Read the model definition and answer for the solid it produces. Units are mm, in the model's axes. Face numbers are marked on the shaded views. Give positions to 0.01 mm unless a question says otherwise; leave off trailing zeros. Order: outer loops, then holes, each group sorted by start corner. A loop starts at its lowest first (then second) coordinate and runs counter-clockwise, first axis right, second up. Notation, with made-up numbers: (64, 22) -> (95, 22) arc R27 ccw to (95, 52) -> close; hole circle Ø3 at (22.25, 17). An arc over 180 degrees is marked (long way). Answer as CSV lines item,"result". Start each with the question number.
1) A flat-ended cylindrical pin translates along its axis: pin 1 Ø16 at (x, y) = (45, 35) entering from +Z. Find the tip coordinate at first contact, or state that the pin passes through.
2) Find section C-C (x = 82). Determine the outline of the cut face in (y, z).
3) Find section D-D (y = 37). Determine the outline of the cut face in (x, z), and give its area (3 significant figures).
4) Find section B-B (y = 65). Determine the outline of the cut face in (x, z), and give its area (3 significant figures).
5) Find section A-A (x = 45). Determine the outline of the cut face in (y, z).
6) Straight lines are drawn through the part: L1, parallel to X at y = 7.5, z = 8; L2, parallel to Y at x = 45, z = 2.45; L3, parallel to Y at x = 45, z = 12.5. For each, find the intervals that lie inside material, in ascending order. Write a range as from..to.
7) The mould has two halves that part along Y. Classify the marked faces 1, 2, 3 and 4: +Y half, -Y half, draft (parallel to the pull), parting line (faces both ways), or undercut.
```python
from build123d import *

# Parameters (mm, degrees)
F0_W           = 90
F0_H           = 15
F4_D           = 8.8
F6_D           = 11
F6_CBORE_D     = 20
F6_CBORE_DEPTH = 12


with BuildPart() as f2:
    # F2: sweep along a path in F1
    with BuildLine(Plane.YZ) as f2_path:
        Line((0, 0), (70, 0))
    # F0 (on Front) → F2 (sweep)
    with BuildSketch(Plane.XZ):
        with Locations((45, 7.5)):
            Rectangle(F0_W, F0_H)
    sweep(path=f2_path.line)

    # F4 (through all)
    with Locations(Plane.XY.offset(15)):
        with Locations((8, 62), (82, 62), (82, 8), (8, 8)):
            Hole(F4_D / 2)

    # F6 (through all)
    with Locations(Plane.XY.offset(15)):
        with Locations((45, 35)):
            CounterBoreHole(F6_D / 2, F6_CBORE_D / 2, F6_CBORE_DEPTH)


solid = f2.part
```
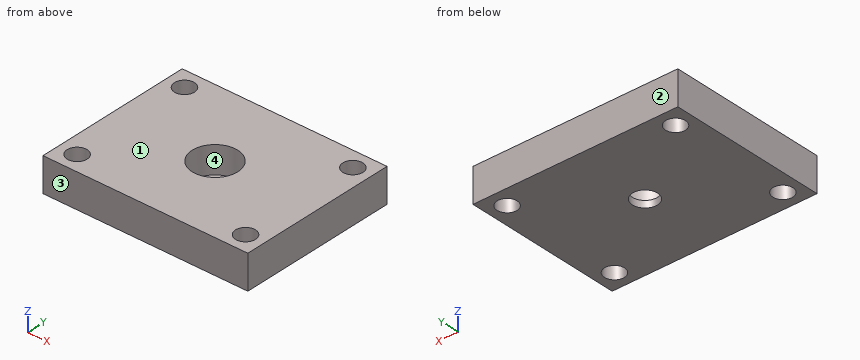
Findings below:
1,pin 1,"z = 3"
2,outline,"(0, 0) -> (3.6, 0) -> (3.6, 15) -> (0, 15) -> close; (12.4, 0) -> (57.6, 0) -> (57.6, 15) -> (12.4, 15) -> close; (66.4, 0) -> (70, 0) -> (70, 15) -> (66.4, 15) -> close"
3,outline,"(0, 0) -> (39.88, 0) -> (39.88, 3) -> (35.2, 3) -> (35.2, 15) -> (0, 15) -> close; (50.12, 0) -> (90, 0) -> (90, 15) -> (54.8, 15) -> (54.8, 3) -> (50.12, 3) -> close"
3,area,"1,080 mm²"
4,outline,"(0, 0) -> (4.78, 0) -> (4.78, 15) -> (0, 15) -> close; (11.22, 0) -> (78.78, 0) -> (78.78, 15) -> (11.22, 15) -> close; (85.22, 0) -> (90, 0) -> (90, 15) -> (85.22, 15) -> close"
4,area,"1,160 mm²"
5,outline,"(0, 0) -> (29.5, 0) -> (29.5, 3) -> (25, 3) -> (25, 15) -> (0, 15) -> close; (40.5, 0) -> (70, 0) -> (70, 15) -> (45, 15) -> (45, 3) -> (40.5, 3) -> close"
6,L1,"0..3.63, 12.37..77.63, 86.37..90"
6,L2,"0..29.5, 40.5..70"
6,L3,"0..25, 45..70"
7,face 1,"draft"
7,face 2,"+Y half"
7,face 3,"-Y half"
7,face 4,"undercut"
